Read the model definition and answer for the solid it produces. Units are mm, in the model's axes. A direction names the side the tool comes from. Coordinates: 2 decimals unless noted, no trailing zeros. Write each loop counter-clockwise with the first axis right and the second up, starting at its lowest first coordinate (ties: lowest second). Pieces come first, ordered by that corner, then holes. Notation, with made-up numbers: M 59.5,47.5 L 110.5,47.5 A19 cw 110.5,70.5 Z; hole C 67,40 d4. An arc over 180 degrees is marked long. Write item = value, one per line.
from build123d import *

# Parameters (mm, degrees)
SKETCH_1_W          = 100
SKETCH_1_H          = 45
EXTRUDE_1_DEPTH     = 2
SKETCH_2_W          = 16
SKETCH_2_H          = 3
EXTRUDE_2_DEPTH     = 10
SKETCH_3_R          = 2.25
CUT_EXTRUDE_1_DEPTH = 111.113577728
SKETCH_4_W          = 5
SKETCH_4_H          = 5
EXTRUDE_3_DEPTH     = 12
FILLET_1_R          = 5
FILLET_2_R          = 5
FILLET_3_R          = 2
SKETCH_5_W          = 1
SKETCH_5_H          = 5.209702161
CUT_EXTRUDE1_DEPTH  = 10


with BuildPart() as part:
    # 草图1 → 凸台-拉伸1 (new body)
    with BuildSketch(Plane(origin=(0, 0, 0), x_dir=(1, 0, 0), z_dir=(0, 1, 0))):
        with Locations((50, -22.5)):
            Rectangle(SKETCH_1_W, SKETCH_1_H)
    extrude(amount=EXTRUDE_1_DEPTH)

    # 草图2 → 凸台-拉伸2 (add)
    with BuildSketch(Plane(origin=(0, 0, 0), x_dir=(-1, 0, 0), z_dir=(0, -1, 0))):
        with Locations((-10, -43.5)):
            Rectangle(SKETCH_2_W, SKETCH_2_H)
        with Locations((-10, -1.5)):
            Rectangle(SKETCH_2_W, SKETCH_2_H)
        with Locations((-90, -43.5)):
            Rectangle(SKETCH_2_W, SKETCH_2_H)
        with Locations((-90, -1.5)):
            Rectangle(SKETCH_2_W, SKETCH_2_H)
    extrude(amount=EXTRUDE_2_DEPTH)

    # 草图3 → 切除-拉伸1 (cut, through all)
    with BuildSketch(Plane.XY.offset(45)):
        with Locations((90, -6)):
            Circle(SKETCH_3_R)
        with Locations((10, -6)):
            Circle(SKETCH_3_R)
    extrude(amount=-CUT_EXTRUDE_1_DEPTH, mode=Mode.SUBTRACT)

    # 草图4 → 凸台-拉伸3 (add)
    with BuildSketch(Plane(origin=(0, 0, 0), x_dir=(-1, 0, 0), z_dir=(0, -1, 0))):
        with Locations((-72.5, -22.5)):
            Rectangle(SKETCH_4_W, SKETCH_4_H)
    extrude(amount=EXTRUDE_3_DEPTH)

    # 圆角1
    fillet_1_edges = [part.edges().sort_by_distance(p)[0] for p in [
        (2, -10, 43.5),
        (18, -10, 43.5),
        (2, -10, 1.5),
        (18, -10, 1.5),
        (82, -10, 43.5),
        (98, -10, 43.5),
        (82, -10, 1.5),
        (98, -10, 1.5),
    ]]
    fillet(fillet_1_edges, radius=FILLET_1_R)

    # 圆角2
    fillet_2_edges = [part.edges().sort_by_distance(p)[0] for p in [
        (70, 0, 22.5),
    ]]
    fillet(fillet_2_edges, radius=FILLET_2_R)
    fillet_2_2_edges = [part.edges().sort_by_distance(p)[0] for p in [
        (70, -12, 22.5),
    ]]
    fillet(fillet_2_2_edges, radius=FILLET_2_R - 0.0001)  # a hair under: the kernel refuses the full size

    # 圆角3
    fillet_3_edges = [part.edges().sort_by_distance(p)[0] for p in [
        (10, 0, 42),
        (10, 0, 3),
        (90, 0, 42),
        (90, 0, 3),
    ]]
    fillet(fillet_3_edges, radius=FILLET_3_R)

    # 草图5 → Cut-Extrude1 (cut)
    with BuildSketch(Plane.XY.offset(25)):
        with Locations((74.5, -6.55317269)):
            Rectangle(SKETCH_5_W, SKETCH_5_H)
    extrude(amount=-CUT_EXTRUDE1_DEPTH, mode=Mode.SUBTRACT)


solid = part.part
Item 1: Consider line 1 along Z through (x, y) = (94.5, -6.25); line 2 along Y through (x, z) = (90, 0.95); line 3 along Y through (x, z) = (95, 7). Determine where each line is inside the solid, lowest interval first. Write a range as from..to.
Worked answers:
line_1 = 0..3, 42..45
line_2 = -10..-8.25, -3.75..2
line_3 = 0..2
Item 2: For a pull along Z with two mould halves and no side action, classify faces 5 (the face through (89.89, -0.57, 3.6)), 6 (the face through (72, -5, 20)), 7 (the face through (18, -2, 1)) as released by +Z, released by -Z, zero draft, split by the parting line, or undercut.
Worked answers:
face_5 = undercut
face_6 = released by -Z
face_7 = zero draft
Item 3: Find section C-C (y = -6). State how many separate pieces and enclosed holes the cut face has, and give its area (3 significant figures).
Worked answers:
separate_pieces = 9
enclosed_holes = 0
area = 156 mm²
Item 4: Which of the six approach directions +Z, -Z, +X, -X, +Y, -Y give full straight-line access (tool end or side, diameter ignored) to faces 1 (the face through (9.89, -0.57, 41.4)), 2 (the face through (2, -2, 44)), 3 (the face through (49, 0, 22)), 4 (the face through (98, -2, 44))?
Worked answers:
face_1 = +X, -X, -Y
face_2 = +Z, -Z, -X, -Y
face_3 = -Y
face_4 = +Z, -Z, +X, -Y
Item 5: Find section D-D (x = 76.5). Determine the outline of the cut face in (y, z), and give its area (3 significant figures).
Worked answers:
outline = M 0,0 L 2,0 L 2,45 L 0,45 Z
area = 90.0 mm²
Item 6: Flat-ended cylindrical pins translate along their axes: pin 1 (8 mm diameter, centred on x = 68.5, y = -4.5, fed in from -Z); pin 2 (6 mm diameter, centred on y = -8.5, z = 5, fed in from -X); pin 3 (2.5 mm diameter, centred on y = -5.5, z = 22, fed in from +X). Find the tip coordinate at first contact, or state that the pin passes through.
Worked answers:
pin_1 = 20
pin_2 = 2.16
pin_3 = 74
Item 7: Find section A-A (x = 10). Determine the outline of the cut face in (y, z), and give its area (3 significant figures).
Worked answers:
outline = M -10,0 L -8.25,0 L -8.25,3 L -10,3 Z; M -10,42 L -8.25,42 L -8.25,45 L -10,45 Z; M -3.75,0 L 2,0 L 2,45 L -3.75,45 L -3.75,42 L -2,42 A2 cw 0,40 L 0,5 A2 cw -2,3 L -3.75,3 Z
area = 125 mm²
